from build123d import *

# Parameters (mm, degrees)
SKETCH_1_W          = 232
SKETCH_1_H          = 52
EXTRUDE_1_DEPTH     = 2
SKETCH_3_R          = 1.55
CUT_EXTRUDE_2_DEPTH = 10
FILLET_1_R          = 3
SKETCH_8_R          = 1.6
CUT_EXTRUDE_6_DEPTH = 10
CUT_EXTRUDE_7_DEPTH = 5
CUT_EXTRUDE_8_DEPTH = 5
FILLET_2_R          = 2


with BuildPart() as part:
    # 草图1 → 凸台-拉伸1 (new body)
    with BuildSketch(Plane.XY):
        Rectangle(SKETCH_1_W, SKETCH_1_H)
    extrude(amount=EXTRUDE_1_DEPTH)

    # 草图3 → 切除-拉伸2 (cut)
    with BuildSketch(Plane.XY.offset(2)):
        with Locations((32, -16)):
            Circle(SKETCH_3_R)
        with Locations((32, 16)):
            Circle(SKETCH_3_R)
        with Locations((-32, 16)):
            Circle(SKETCH_3_R)
        with Locations((-32, -16)):
            Circle(SKETCH_3_R)
    extrude(amount=-CUT_EXTRUDE_2_DEPTH, mode=Mode.SUBTRACT)

    # 圆角1
    fillet_1_edges = [part.edges().sort_by_distance(p)[0] for p in [
        (116, -26, 1),
        (-116, -26, 1),
        (-116, 26, 1),
        (116, 26, 1),
    ]]
    fillet(fillet_1_edges, radius=FILLET_1_R)

    # 草图8 → 切除-拉伸6 (cut)
    with BuildSketch(Plane.XY.offset(2)):
        with Locations((-106, 15)):
            Circle(SKETCH_8_R)
        with Locations((-106, -15)):
            Circle(SKETCH_8_R)
    cut_extrude_6 = extrude(amount=-CUT_EXTRUDE_6_DEPTH, mode=Mode.SUBTRACT)

    # 镜向1: 切除-拉伸6 across plane
    add(cut_extrude_6.mirror(Plane(origin=(0, 0, 0), x_dir=(0, 0, 1), z_dir=(1, 0, 0))), mode=Mode.SUBTRACT)

    # 草图9 → 切除-拉伸7 (cut, symmetric)
    with BuildSketch(Plane.XY.offset(2)):
        with BuildLine():
            ThreePointArc((-116, -23), (-115.121320344, -25.121320344), (-113, -26))
            Line((-113, -26), (113, -26))
            ThreePointArc((113, -26), (115.121320344, -25.121320344), (116, -23))
            Line((116, -23), (116, 23))
            ThreePointArc((116, 23), (115.121320344, 25.121320344), (113, 26))
            Line((113, 26), (-113, 26))
            ThreePointArc((-113, 26), (-115.121320344, 25.121320344), (-116, 23))
            Line((-116, 23), (-116, -23))
        make_face()
        with BuildLine():
            Line((-110, -15), (-110, 15))
            ThreePointArc((-110, 15), (-108.847472254, 17.809252883), (-106.054049119, 18.99963482))
            Line((-106.054049119, 18.99963482), (-32.054049119, 19.99963482))
            ThreePointArc((-32.054049119, 19.99963482), (-32.027025176, 19.999908704), (-32, 20))
            Line((-32, 20), (32, 20))
            ThreePointArc((32, 20), (32.027025176, 19.999908704), (32.054049119, 19.99963482))
            Line((32.054049119, 19.99963482), (106.054049119, 18.99963482))
            ThreePointArc((106.054049119, 18.99963482), (108.847472254, 17.809252883), (110, 15))
            Line((110, 15), (110, -15))
            ThreePointArc((110, -15), (108.847472254, -17.809252883), (106.054049119, -18.99963482))
            Line((106.054049119, -18.99963482), (32.054049119, -19.99963482))
            ThreePointArc((32.054049119, -19.99963482), (32.027025176, -19.999908704), (32, -20))
            Line((32, -20), (-32, -20))
            ThreePointArc((-32, -20), (-32.027025176, -19.999908704), (-32.054049119, -19.99963482))
            Line((-32.054049119, -19.99963482), (-106.054049119, -18.99963482))
            ThreePointArc((-106.054049119, -18.99963482), (-108.847472254, -17.809252883), (-110, -15))
        make_face(mode=Mode.SUBTRACT)
    extrude(amount=CUT_EXTRUDE_7_DEPTH, both=True, mode=Mode.SUBTRACT)

    # 草图10 → 切除-拉伸8 (cut, symmetric)
    with BuildSketch(Plane.XY.offset(2)):
        Polygon((-70.226242813, 1.607711368), (-38.319534037, 13.914418285), (-99.972894719, 13.081264762), align=None)
        Polygon((-104, -11.419133052), (-74.394439777, 0), (-104, 11.419133052), align=None)
        Polygon((-38.319534037, -13.914418285), (-70.226242813, -1.607711368), (-99.972894719, -13.081264762), align=None)
        Polygon((-34, -12.365078998), (-34, 12.365078998), (-66.058045849, 0), align=None)
        Polygon((-30, -12.344705464), (-3.547059719, 0), (-30, 12.344705464), align=None)
        Polygon((-26.452940281, 14), (0, 1.655294536), (26.452940281, 14), align=None)
        Polygon((3.547059719, 0), (30, -12.344705464), (30, 12.344705464), align=None)
        Polygon((34, -12.365078998), (66.058045849, 0), (34, 12.365078998), align=None)
        Polygon((70.226242813, 1.607711368), (99.972894719, 13.081264762), (38.319534037, 13.914418285), align=None)
        Polygon((104, 11.419133052), (74.394439777, 0), (104, -11.419133052), align=None)
        Polygon((99.972894719, -13.081264762), (70.226242813, -1.607711368), (38.319534037, -13.914418285), align=None)
        Polygon((-26.452940281, -14), (26.452940281, -14), (0, -1.655294536), align=None)
    extrude(amount=CUT_EXTRUDE_8_DEPTH, both=True, mode=Mode.SUBTRACT)

    # 圆角2
    fillet_2_edges = [part.edges().sort_by_distance(p)[0] for p in [
        (34, -12.365078998, 1),
        (34, 12.365078998, 1),
        (66.058045849, 0, 1),
        (38.319534037, 13.914418285, 1),
        (99.972894719, 13.081264762, 1),
        (70.226242813, 1.607711368, 1),
        (26.452940281, 14, 1),
        (0, 1.655294536, 1),
        (-26.452940281, 14, 1),
        (30, 12.344705464, 1),
        (30, -12.344705464, 1),
        (3.547059719, 0, 1),
        (-70.226242813, -1.607711368, 1),
        (-38.319534037, -13.914418285, 1),
        (-99.972894719, -13.081264762, 1),
        (-104, -11.419133052, 1),
        (-104, 11.419133052, 1),
        (-74.394439777, 0, 1),
        (-66.058045849, 0, 1),
        (-34, 12.365078998, 1),
        (-34, -12.365078998, 1),
        (-3.547059719, 0, 1),
        (-30, -12.344705464, 1),
        (-30, 12.344705464, 1),
        (99.972894719, -13.081264762, 1),
        (38.319534037, -13.914418285, 1),
        (70.226242813, -1.607711368, 1),
        (104, 11.419133052, 1),
        (104, -11.419133052, 1),
        (74.394439777, 0, 1),
        (0, -1.655294536, 1),
        (26.452940281, -14, 1),
        (-26.452940281, -14, 1),
        (-99.972894719, 13.081264762, 1),
        (-38.319534037, 13.914418285, 1),
        (-70.226242813, 1.607711368, 1),
    ]]
    fillet(fillet_2_edges, radius=FILLET_2_R)


solid = part.part
CAD build for the part. Positions are in the model's coordinates, mm. A direction names the side the tool comes from. Give positions to 0.01 mm unless a question says otherwise; leave off trailing zeros. Answer in a Markdown table with one row per item.
1. Tool access for faces 4 (the flat face through (-9.687, 6.176, 0.986)), 5 (the flat face through (-2, 0, 0)): list every direction of +Z, -Z, +X, -X, +Y, -Y with a clear straight run to the whole face (end or side of a thin tool).
Data:
| item | result |
|---|---|
| face 4 | +Z, -Z |
| face 5 | -Z, +X, -X, +Y, -Y |
2. Probe probe 1 along Y at (x, z) = (-32, 0.9); probe 2 along Y at (x, z) = (106, 1.15); probe 3 along Y at (x, z) = (16, 0.1). List the from-to ranges inside material, lowest first. Write a range as [from, to].
Data:
| item | result |
|---|---|
| probe 1 | y = [-20, -17.55], [-14.45, 14.45], [17.55, 20] |
| probe 2 | y = [-19, -16.6], [-13.4, 13.4], [16.6, 19] |
| probe 3 | y = [-20, -14], [-9.12, -5.81], [5.81, 9.12], [14, 20] |
3. Flat gauge pin, fed straight in: pin 1 (12 mm diameter, centred on x = 0.5, y = -14.5, fed in from -Z). Where does the tip first touch, or does it go through?
Data:
| item | result |
|---|---|
| pin 1 | stops at z = 0 |
4. Saw through at A-A, the plane z = 1. Count the separate pieces of the cut face and the enclosed holes in it, plus the area to 3 significant figures.
Data:
| item | result |
|---|---|
| separate pieces | 1 |
| enclosed holes | 20 |
| area | 4,550 mm² |
5. Pull direction Y, two halves, no side cores. Call faces 1 (the flat face through (-17.43, -6.48, 0.99)), 2 (the cylindrical face through (108.817, 17.84, 1.014)), 3 (the cylindrical face through (-108.817, -17.84, 1.014)): pulls with the +Y half, pulls with the -Y half, needs draft (parallel to the pull), parting line crosses it, or undercut.
Data:
| item | result |
|---|---|
| face 1 | undercut |
| face 2 | pulls with the +Y half |
| face 3 | pulls with the -Y half |
